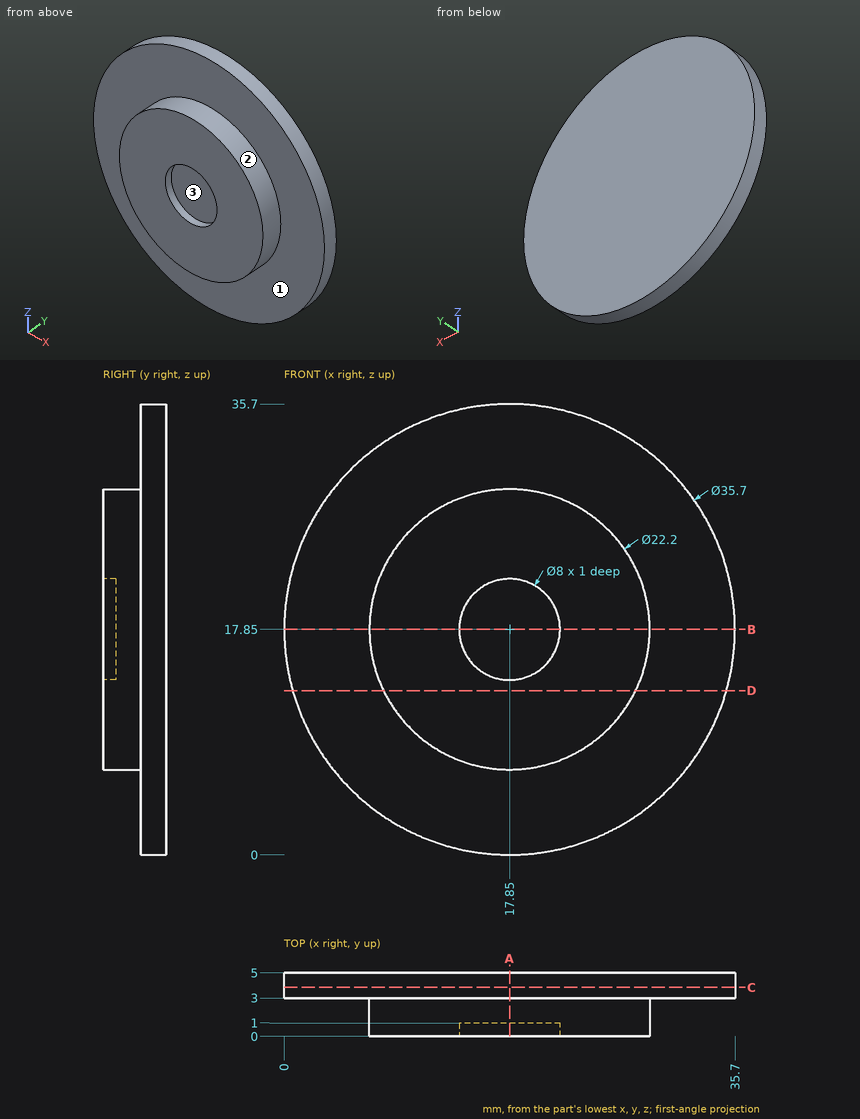
The drawing under review shows one solid part. Ordinate dimensions are in mm from its lowest x, y, z. Round coordinates to 2 decimals unless told otherwise and drop trailing zeros. Write each loop counter-clockwise with the first axis right and the second up, starting at its lowest first coordinate (ties: lowest second). Pieces come first, ordered by that corner, then holes. Notation, with made-up numbers: (57.25, 3) - (96.25, 3) arc R10 cw to (96.25, 8) - close; hole circle Ø10 at (81, -16.75). An arc over 180 degrees is marked (long way). Write each question's results on one line, items separated by ' | '.
Item 1: To check wall thickness, follow line 1 along Z through (x, y) = (17.85, 0.2); line 2 along Y through (x, z) = (10, 8); line 3 along Z through (x, y) = (19, 0.75). State the ranges of each line that lie inside material, in increasing order. Write a range as from..to.
Calculated:
line 1: z = 6.75..13.85, 21.85..28.95 | line 2: y = 3..5 | line 3: z = 6.81..14.02, 21.68..28.89
Item 2: For pin 1 (1 mm diameter, centred on x = 7.5, y = 2, fed in from +Z); pin 2 (2.5 mm diameter, centred on x = 16.5, z = 18, fed in from -Y); pin 3 (1.5 mm diameter, centred on x = 8, y = 1.5, fed in from -Z), all flat-tipped, find the tip position at first contact; note any pin that passes through.
Calculated:
pin 1: stops at z = 22.97 | pin 2: stops at y = 1 | pin 3: stops at z = 11.49
Item 3: Take a section at C-C on y = 3.85. State the section outline as (x, z) points, then the cut area to 3 significant figures.
Calculated:
outline: circle Ø35.7 at (17.85, 17.85) | area: 1,000 mm^2
Item 4: Take a section at D-D on z = 13. State the section outline as (x, y) points.
Calculated:
outline: (0.67, 3) - (7.87, 3) - (7.87, 0) - (27.83, 0) - (27.83, 3) - (35.03, 3) - (35.03, 5) - (0.67, 5) - close
Item 5: Draft analysis for pull direction X (two halves, no side actions). For the marked faces 1, 2 and 3, state which applies: pulls with the +X half, pulls with the -X half, needs draft (parallel to the pull), parting line crosses it, or undercut.
Calculated:
face 1: needs draft | face 2: parting line crosses it | face 3: undercut
Item 6: Take a section at A-A on x = 17.85. State the section outline as (y, z) points, then the cut area to 3 significant figures.
Calculated:
outline: (0, 6.75) - (3, 6.75) - (3, 0) - (5, 0) - (5, 35.7) - (3, 35.7) - (3, 28.95) - (0, 28.95) - (0, 21.85) - (1, 21.85) - (1, 13.85) - (0, 13.85) - close | area: 130 mm^2
Item 7: Take a section at B-B on z = 17.85. State the section outline as (x, y) points.
Calculated:
outline: (0, 3) - (6.75, 3) - (6.75, 0) - (13.85, 0) - (13.85, 1) - (21.85, 1) - (21.85, 0) - (28.95, 0) - (28.95, 3) - (35.7, 3) - (35.7, 5) - (0, 5) - close
